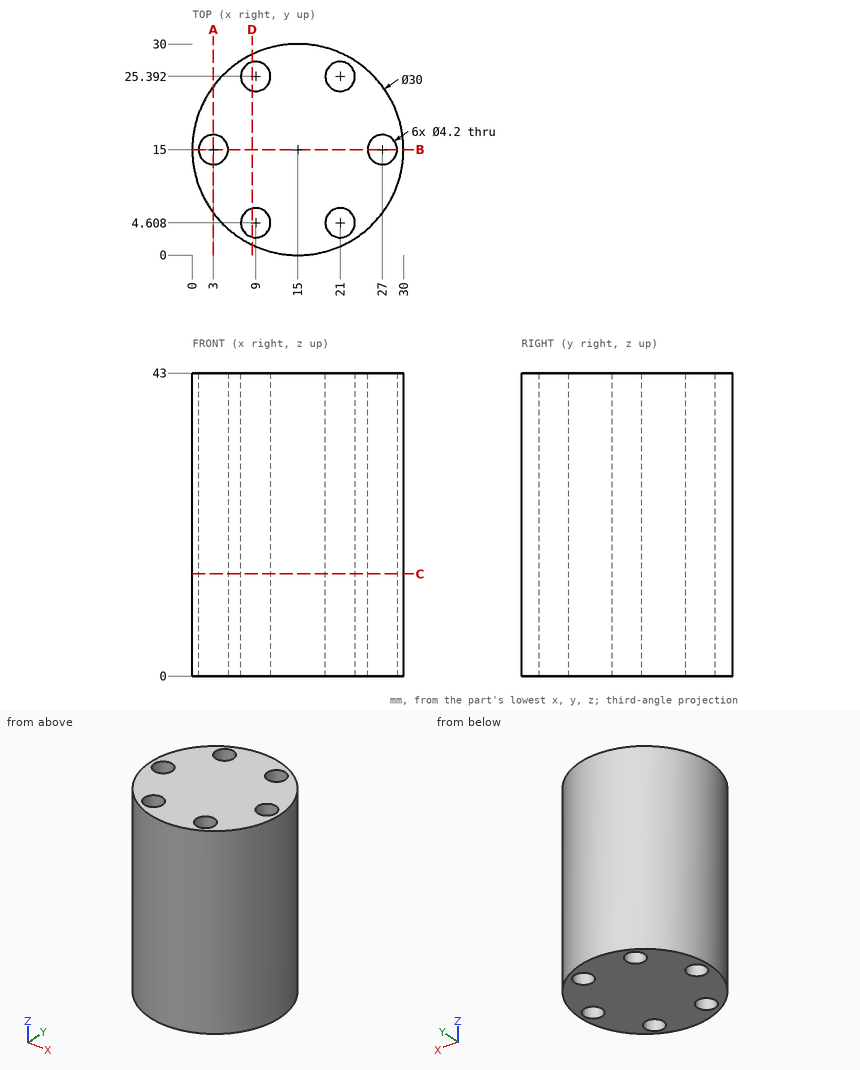
Check sheet for the drawn part. Datum: minimum x, y, z corner. Units: mm. Coordinates: 2 decimals unless noted, no trailing zeros. Order: outer loops, then holes, each group sorted by start corner. A loop starts at its lowest first (then second) coordinate and runs counter-clockwise, first axis right, second up. Notation, with made-up numbers: (32, -4) -> (52, -4) arc R15 cw to (52, 22) -> close; hole circle Ø9 at (43, 35.25). An arc over 180 degrees is marked (long way). Use a Markdown table: item, result. Add a question column.
1. Cross-section at D-D (x = 8.5). Enter the section's corners in (y, z), and give its area (3 significant figures).
2. Cross-section at C-C (z = 14.5). Enter the section's corners in (x, y), and give its area (3 significant figures).
3. Cross-section at B-B (y = 15). Enter the section's corners in (x, z).
4. Go/stop test with flat-tipped pins: pin 1 Ø1 at (y, z) = (19, 34) entering from -X; pin 2 Ø6 at (x, y) = (18.5, 6) entering from -Z; pin 3 Ø2 at (x, z) = (20, 6) entering from +Y; pin 4 Ø3 at (y, z) = (24, 10) entering from -X. Record where each tip stops, or that it passes through.
5. Material ranges on L1, parallel to X at y = 5, z = 17; L2, parallel to Y at x = 9, z = 14.5; L3, parallel to X at y = 16.5, z = 8.5 (1 decimal), recorded low to high.
6. Cross-section at A-A (x = 3). Enter the section's corners in (y, z).
Filled sheet:
| question | item | result |
|---|---|---|
| 1 | outline | (1.48, 0) -> (2.57, 0) -> (2.57, 43) -> (1.48, 43) -> close; (6.65, 0) -> (23.35, 0) -> (23.35, 43) -> (6.65, 43) -> close; (27.43, 0) -> (28.52, 0) -> (28.52, 43) -> (27.43, 43) -> close |
| 1 | area | 812 mm2 |
| 2 | outline | circle Ø30 at (15, 15); hole circle Ø4.2 at (3, 15); hole circle Ø4.2 at (9, 4.61); hole circle Ø4.2 at (9, 25.39); hole circle Ø4.2 at (21, 4.61); hole circle Ø4.2 at (21, 25.39); hole circle Ø4.2 at (27, 15) |
| 2 | area | 624 mm2 |
| 3 | outline | (0, 0) -> (0.9, 0) -> (0.9, 43) -> (0, 43) -> close; (5.1, 0) -> (24.9, 0) -> (24.9, 43) -> (5.1, 43) -> close; (29.1, 0) -> (30, 0) -> (30, 43) -> (29.1, 43) -> close |
| 4 | pin 1 | x = 0.41 |
| 4 | pin 2 | z = 0 |
| 4 | pin 3 | y = 29.46 |
| 4 | pin 4 | x = 2.01 |
| 5 | L1 | 3.82 to 6.94, 11.06 to 18.94, 23.06 to 26.18 |
| 5 | L2 | 1.25 to 2.51, 6.71 to 23.29, 27.49 to 28.75 |
| 5 | L3 | 0.1 to 1.5, 4.5 to 25.5, 28.5 to 29.9 |
| 6 | outline | (6, 0) -> (12.9, 0) -> (12.9, 43) -> (6, 43) -> close; (17.1, 0) -> (24, 0) -> (24, 43) -> (17.1, 43) -> close |
